Design review of the part shown in the three views and the two pictorial views. Dimensions are in mm from the part's minimum x, y and z. A direction names the side the tool comes from. Round coordinates to 2 decimals unless told otherwise and drop trailing zeros. Write each loop counter-clockwise with the first axis right and the second up, starting at its lowest first coordinate (ties: lowest second). Pieces come first, ordered by that corner, then holes. Notation, with made-up numbers: (17.25, 74.5) -> (22.25, 74.5) arc R10 ccw to (22.25, 82.5) -> close; hole circle Ø5 at (54, 16.25). An arc over 180 degrees is marked (long way). Answer as a JSON object with one key per item and string values. Group by question number.
1) We need section D-D, the plane x = 16.1. Write out the cut boundary in (y, z).
2) We need section C-C, the plane y = 53.5. Write out the cut boundary in (x, z).
3) To check wall thickness, follow probe 1 along Y at (x, z) = (26.4, 21.2); probe 2 along X at (y, z) = (34, 23.5); probe 3 along X at (y, z) = (68, 6.5). State the ranges of each line that lie inside material, in increasing order. Write a range as [from, to].
4) Insertion check: pin 1 Ø4 at (y, z) = (20, 17) entering from -X; pin 2 Ø4 at (y, z) = (31, 16.5) entering from +X; pin 3 Ø3 at (x, z) = (26, 20.5) entering from +Y; pin 4 Ø2.5 at (x, y) = (16.1, 53.5) entering from -Z. Each pin has a flat end and moves straight along its axis. Give the tip position at first contact, or say it passes through.
5) Mouldability with a two-part tool opening along Y and no side actions: class the marked faces 5, 6 and 7 as pulls with the +Y half, pulls with the -Y half, needs draft (parallel to the pull), parting line crosses it, or undercut.
6) Machinability: for the marked faces 1, 2, 3 and 4, which of the approach directions +Z, -Z, +X, -X, +Y, -Y give a long, thin tool a straight path to every point of the face, cutting with its end or side? Answer none if there is none.
7) We need section B-B, the plane z = 12.5. Count the separate pieces of the cut face and the enclosed holes in it, then the cut area to 3 significant figures.
8) We need section A-A, the plane y = 70. Write out the cut boundary in (x, z).
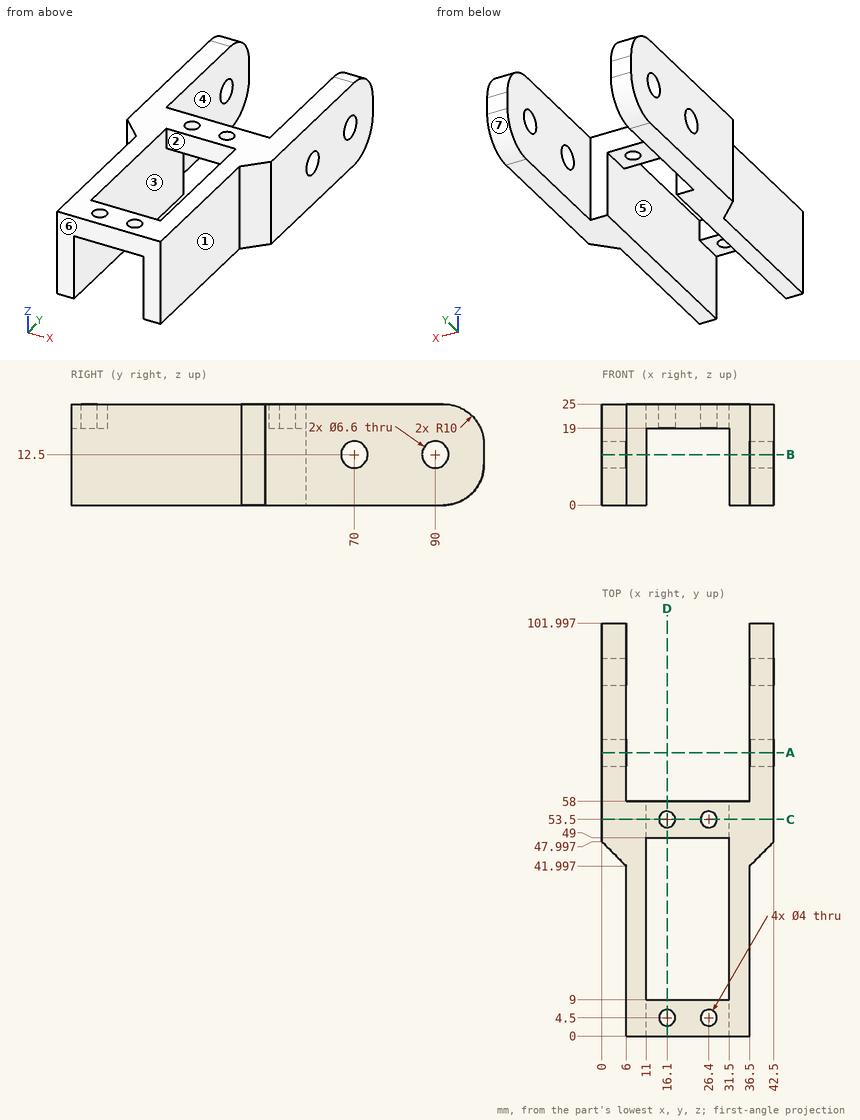
Here are the results:
{
 "1": {"outline": "(0, 19) -> (2.5, 19) -> (2.5, 25) -> (0, 25) -> close; (6.5, 19) -> (9, 19) -> (9, 25) -> (6.5, 25) -> close; (49, 19) -> (51.5, 19) -> (51.5, 25) -> (49, 25) -> close; (55.5, 19) -> (58, 19) -> (58, 25) -> (55.5, 25) -> close"},
 "2": {"outline": "(0, 0) -> (11, 0) -> (11, 19) -> (14.1, 19) -> (14.1, 25) -> (0, 25) -> close; (18.1, 19) -> (24.4, 19) -> (24.4, 25) -> (18.1, 25) -> close; (28.4, 19) -> (31.5, 19) -> (31.5, 0) -> (42.5, 0) -> (42.5, 25) -> (28.4, 25) -> close"},
 "3": {"probe 1": "y = [0, 2.5], [6.5, 9], [49, 51.5], [55.5, 58]", "probe 2": "x = [6, 11], [31.5, 36.5]", "probe 3": "x = [0, 6], [36.5, 42.5]"},
 "4": {"pin 1": "stops at x = 6", "pin 2": "stops at x = 36.5", "pin 3": "stops at y = 58", "pin 4": "passes through"},
 "5": {"face 5": "undercut", "face 6": "pulls with the -Y half", "face 7": "pulls with the +Y half"},
 "6": {"face 1": "+Z, -Z, +X, -Y", "face 2": "+Z, -Z", "face 3": "-Z", "face 4": "+Z, -Z, +Y"},
 "7": {"separate pieces": "6", "enclosed holes": "0", "area": "1,110 mm^2"},
 "8": {"outline": "(0, 0) -> (6, 0) -> (6, 9.2) -> (0, 9.2) -> close; (0, 15.8) -> (6, 15.8) -> (6, 25) -> (0, 25) -> close; (36.5, 0) -> (42.5, 0) -> (42.5, 9.2) -> (36.5, 9.2) -> close; (36.5, 15.8) -> (42.5, 15.8) -> (42.5, 25) -> (36.5, 25) -> close"}
}
